from build123d import *

# Parameters (mm, degrees)
SKETCH1_R           = 26
SKETCH1_R_2         = 14
BOSS_EXTRUDE1_DEPTH = 8
BOSS_EXTRUDE2_DEPTH = 8
SKETCH3_W           = 12.5
SKETCH3_H           = 2
SKETCH4_W           = 1.3
SKETCH4_H           = 0.7
SKETCH5_W           = 16
SKETCH5_H           = 45.261366246
BOSS_EXTRUDE3_DEPTH = 8
FILLET1_R           = 10
SKETCH6_R           = 3
CUT_EXTRUDE1_DEPTH  = 125.9799984
SKETCH9_R           = 6.5
CUT_EXTRUDE4_DEPTH  = 7
SKETCH10_R          = 3
CUT_EXTRUDE5_DEPTH  = 124.822453537


with BuildPart() as part:
    # Sketch1 → Boss-Extrude1 (new, symmetric)
    with BuildSketch(Plane.XY):
        Circle(SKETCH1_R)
        Circle(SKETCH1_R_2, mode=Mode.SUBTRACT)
    extrude(amount=BOSS_EXTRUDE1_DEPTH, both=True)

    # Sketch2 → Boss-Extrude2 (add, symmetric)
    with BuildSketch(Plane.XY):
        Polygon((-8, 120), (8, 120), (8, 24.738633754), (0, 26), (-8, 24.738633754), align=None)
    extrude(amount=BOSS_EXTRUDE2_DEPTH, both=True)

    # Sketch3 → Cut-Revolve1 (revolve, cut)
    with BuildSketch(Plane(origin=(0, 0, 0), x_dir=(0, 0, -1), z_dir=(1, 0, 0)), mode=Mode.PRIVATE) as cut_revolve1_sk:
        with Locations((-1.75, 15)):
            Rectangle(SKETCH3_W, SKETCH3_H)
    revolve(cut_revolve1_sk.sketch.rotate(Axis((0, 0, 0), (0, 0, -1)), 90), axis=Axis((0, 0, 0), (0, 0, -1)), mode=Mode.SUBTRACT)

    # Sketch4 → Cut-Revolve2 (revolve, cut)
    with BuildSketch(Plane(origin=(0, 0, 0), x_dir=(0, 0, -1), z_dir=(1, 0, 0)), mode=Mode.PRIVATE) as cut_revolve2_sk:
        with Locations((-5.05, 16.35)):
            Rectangle(SKETCH4_W, SKETCH4_H)
    revolve(cut_revolve2_sk.sketch.rotate(Axis((0, 0, 0), (0, 0, -1)), 90), axis=Axis((0, 0, 0), (0, 0, -1)), mode=Mode.SUBTRACT)

    # Sketch5 → Boss-Extrude3 (add, symmetric)
    with BuildSketch(Plane.XY):
        with Locations((0, -47.369316877)):
            Rectangle(SKETCH5_W, SKETCH5_H)
    extrude(amount=BOSS_EXTRUDE3_DEPTH, both=True)

    # Fillet1
    fillet1_edges = [part.edges().sort_by_distance(p)[0] for p in [
        (8, 24.738633754, 0),
        (-8, 24.738633754, 0),
        (8, -24.738633754, 0),
        (-8, -24.738633754, 0),
    ]]
    fillet(fillet1_edges, radius=FILLET1_R)

    # Sketch6 → Cut-Extrude1 (cut, through all)
    with BuildSketch(Plane.ZY.offset(8)):
        with Locations(Location((0, 110, 0), (0, 0, 270))):
            Circle(SKETCH6_R)
        with Locations(Location((0, 90, 0), (0, 0, 270))):
            Circle(SKETCH6_R)
    extrude(amount=-CUT_EXTRUDE1_DEPTH, mode=Mode.SUBTRACT)

    # Sketch9 → Cut-Extrude4 (cut)
    with BuildSketch(Plane.XY.offset(8)):
        with Locations((0, -55)):
            Circle(SKETCH9_R)
        with Locations((0, -30)):
            Circle(SKETCH9_R)
    cut_extrude4 = extrude(amount=-CUT_EXTRUDE4_DEPTH, mode=Mode.SUBTRACT)

    # Sketch10 → Cut-Extrude5 (cut, through all)
    with BuildSketch(Plane.XY.offset(8)):
        with Locations((0, -30)):
            Circle(SKETCH10_R)
        with Locations((0, -55)):
            Circle(SKETCH10_R)
    cut_extrude5 = extrude(amount=-CUT_EXTRUDE5_DEPTH, mode=Mode.SUBTRACT)

    # Mirror1: Cut-Extrude4 across plane
    add(cut_extrude4.mirror(Plane.ZX), mode=Mode.SUBTRACT)

    # Mirror2: Cut-Extrude5 across plane
    add(cut_extrude5.mirror(Plane.ZX), mode=Mode.SUBTRACT)


solid = part.part
Could you check a few things on this model? Use its own coordinates, in mm. A direction names the side the tool comes from. Give positions to 0.01 mm unless a question says otherwise; leave off trailing zeros. Order: outer loops, then holes, each group sorted by start corner. A loop starts at its lowest first (then second) coordinate and runs counter-clockwise, first axis right, second up. Notation, with made-up numbers: (-39, 24.25) - (-13, 24.25) arc R22 cw to (-13, 41.25) - close; hole circle Ø2 at (17.25, -23). An arc over 180 degrees is marked (long way). One line per item, written item: value. Start each with the question number.
1. Imagine slicing it at C-C on y = -55. List the corners of the cut face in (x, z) for me.
2. Imagine slicing it at D-D on y = 81. List the corners of the cut face in (x, z) for me.
3. If I drill on probe 1 along Y at (x, z) = (0, 4); probe 2 along X at (y, z) = (55, 3.75); probe 3 along X at (y, z) = (82, 6.75), over which ranges is the centre line in solid material (lowest first)?
4. For faces 4 (the face through (-8, -51, 0)), 5 (the face through (8, -51, 0)), 6 (the face through (-1.409, 61.345, 4.549)), 7 (the face through (8, 76, 0)), which set-ups out of +Z, -Z, +X, -X, +Y, -Y let a thin tool reach every point of the face, with its end or its side?
5. Imagine slicing it at B-B on x = 0. Give the number of separate pieces and of enclosed holes in the cut face, plus the area to 3 significant figures.
6. Imagine slicing it at A-A on y = 0. List the corners of the cut face in (x, z) for me, plus the area to 3 significant figures.
7. For P1, Ø16.5, axis at x = -8.5, y = 4, coming from the -Z side; P2, Ø1, axis at x = -15, z = -2, coming from the -Y side; P3, Ø5, axis at y = 69.5, z = 1.5, coming from the +X side; P4, Ø5.5, axis at y = 110, z = 0, coming from the +X side, each with a flat end and sliding along its axis, tell me the tip position at first contact or that it passes through.
8. Thinking about a two-plate mould opening in Z: for faces 1 (the face through (-9.303, -26.241, -0.112)), 2 (the face through (-2.17, -16.56, 5.04)), 3 (the face through (0.07, 14.15, -4.5)), which applies, +Z half, -Z half, draft (parallel to the pull), parting line (faces both ways), or undercut?
Values:
1. outline: (-8, -8) - (-3, -8) - (-3, 1) - (-6.5, 1) - (-6.5, 8) - (-8, 8) - close; (3, -8) - (8, -8) - (8, 8) - (6.5, 8) - (6.5, 1) - (3, 1) - close
2. outline: (-8, -8) - (8, -8) - (8, 8) - (-8, 8) - close
3. probe 1: -70 to -61.5, -48.5 to -36.5, -23.5 to -16, 16 to 23.5, 36.5 to 48.5, 61.5 to 120
3. probe 2: -8 to -6.5, 6.5 to 8
3. probe 3: -8 to 8
4. face 4: +Z, -Z, -X, -Y
4. face 5: +Z, -Z, +X, -Y
4. face 6: +Z
4. face 7: +Z, -Z, +X, +Y
5. separate pieces: 6
5. enclosed holes: 2
5. area: 1,900 mm²
6. outline: (-26, -8) - (-14, -8) - (-14, -4.5) - (-16, -4.5) - (-16, 4.4) - (-16.7, 4.4) - (-16.7, 5.7) - (-16, 5.7) - (-16, 8) - (-26, 8) - close; (14, -8) - (26, -8) - (26, 8) - (16, 8) - (16, 5.7) - (16.7, 5.7) - (16.7, 4.4) - (16, 4.4) - (16, -4.5) - (14, -4.5) - close
6. area: 332 mm²
7. P1: z = -8
7. P2: y = -21.58
7. P3: x = 8
7. P4: through
8. face 1: draft
8. face 2: undercut
8. face 3: +Z half
